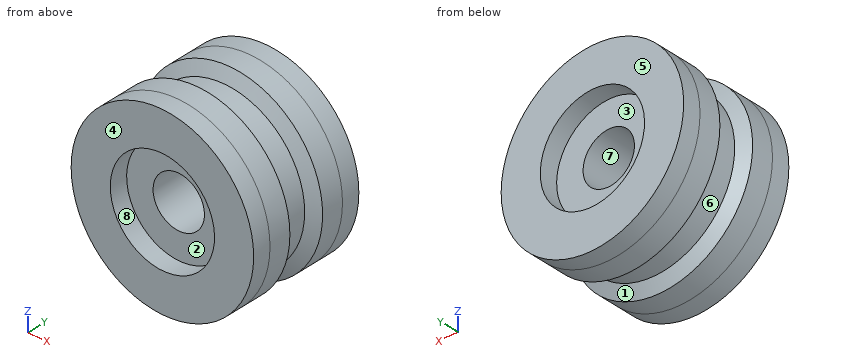
from build123d import *

# Parameters (mm, degrees)
CROQUIS1_R              = 35
CROQUIS1_R_2            = 9.85
SALIENTE_EXTRUIR1_DEPTH = 15.5
CROQUIS3_W              = 15
CROQUIS3_H              = 7


with BuildPart() as part:
    # Croquis1 → Saliente-Extruir1 (new, symmetric)
    with BuildSketch(Plane(origin=(0, 0, 0), x_dir=(1, 0, 0), z_dir=(0, 1, 0))):
        with Locations(Location((0, 0, 0), (0, 0, 270))):
            Circle(CROQUIS1_R)
        with Locations(Location((0, 0, 0), (0, 0, 270))):
            Circle(CROQUIS1_R_2, mode=Mode.SUBTRACT)
    extrude(amount=SALIENTE_EXTRUIR1_DEPTH, both=True)

    # Croquis2 → Cortar-Revolución1 (revolve, cut)
    with BuildSketch(Plane(origin=(0, 0, 0), x_dir=(0, 0, -1), z_dir=(1, 0, 0))):
        Polygon((-30.36, -4.5), (-35, -7), (-35, 7), (-30.36, 4.5), align=None)
    revolve(axis=Axis((0, 15.5, 0), (0, -1, 0)), mode=Mode.SUBTRACT)

    # Croquis3 → Revolución1 (revolve)
    with BuildSketch(Plane(origin=(0, 0, 0), x_dir=(0, 0, -1), z_dir=(1, 0, 0))):
        with Locations((-27.5, 19)):
            Rectangle(CROQUIS3_W, CROQUIS3_H)
        with Locations((-27.5, -19)):
            Rectangle(CROQUIS3_W, CROQUIS3_H)
    revolve(axis=Axis((0, 15.5, 0), (0, -1, 0)))


solid = part.part
Part model, mm, in its own coordinate system. Face numbers are marked on the shaded views. A direction names the side the tool comes from. Round coordinates to 2 decimals unless told otherwise and drop trailing zeros. Write each loop counter-clockwise with the first axis right and the second up, starting at its lowest first coordinate (ties: lowest second). Pieces come first, ordered by that corner, then holes. Notation, with made-up numbers: M -15.5,81.25 L 41.5,81.25 A15 cw 41.5,104.25 Z; hole C -18,24 d11. An arc over 180 degrees is marked long. Return JSON: item names as keys, results as strings. Group by question number.
(1) Drill centre lines: probe 1 along X at (y, z) = (-17.25, 0); probe 2 along Z at (x, y) = (-2.5, -0.5). Where is each one in solid material? Low to high.
(2) Which spindle directions (+Z, -Z, +X, -X, +Y, -Y) get a long thin tool onto all of the face, cutting with end or side? Do the marked faces 1, 2, 3 and 4. Say none if no direction does.
(3) Pin check, flat tips, straight feed: pin 1 Ø12 at (x, z) = (-4, 5.5) entering from -Y; pin 2 Ø8 at (y, z) = (15.5, 5) entering from -X; pin 3 Ø3 at (y, z) = (3.5, -12.5) entering from +X. Stop position of each tip, or through.
(4) Saw through at C-C on y = 8. Write the cut outline in (x, z), then the cut area to 3 significant figures.
(5) Saw through at A-A on z = 0. Write the cut outline in (x, y), then the cut area to 3 significant figures.
(6) Two-plate mould, pull along X, no slides. Class the marked faces 5, 6, 7 and 8: +X half, -X half, draft (parallel to the pull), parting line (faces both ways), or undercut.
(7) Saw through at B-B on x = 0. Write the cut outline in (y, z), then the cut area to 3 significant figures.
Returned:
{
 "1": {"probe 1": "-35 to -20, 20 to 35", "probe 2": "-30.26 to -9.53, 9.53 to 30.26"},
 "2": {"face 1": "none", "face 2": "-Y", "face 3": "+Y", "face 4": "+Z, -Z, +X, -X, -Y"},
 "3": {"pin 1": "y = -15.5", "pin 2": "x = -34.99", "pin 3": "x = 28.75"},
 "4": {"outline": "C 0,0 d70; hole C 0,0 d19.7", "area": "3,540 mm²"},
 "5": {"outline": "M -35,-22.5 L -20,-22.5 L -20,-15.5 L -9.85,-15.5 L -9.85,15.5 L -20,15.5 L -20,22.5 L -35,22.5 L -35,7 L -30.36,4.5 L -30.36,-4.5 L -35,-7 Z; M 9.85,-15.5 L 20,-15.5 L 20,-22.5 L 35,-22.5 L 35,-7 L 30.36,-4.5 L 30.36,4.5 L 35,7 L 35,22.5 L 20,22.5 L 20,15.5 L 9.85,15.5 Z", "area": "1,870 mm²"},
 "6": {"face 5": "draft", "face 6": "parting line", "face 7": "undercut", "face 8": "undercut"},
 "7": {"outline": "M -22.5,-35 L -7,-35 L -4.5,-30.36 L 4.5,-30.36 L 7,-35 L 22.5,-35 L 22.5,-20 L 15.5,-20 L 15.5,-9.85 L -15.5,-9.85 L -15.5,-20 L -22.5,-20 Z; M -22.5,20 L -15.5,20 L -15.5,9.85 L 15.5,9.85 L 15.5,20 L 22.5,20 L 22.5,35 L 7,35 L 4.5,30.36 L -4.5,30.36 L -7,35 L -22.5,35 Z", "area": "1,870 mm²"}
}
